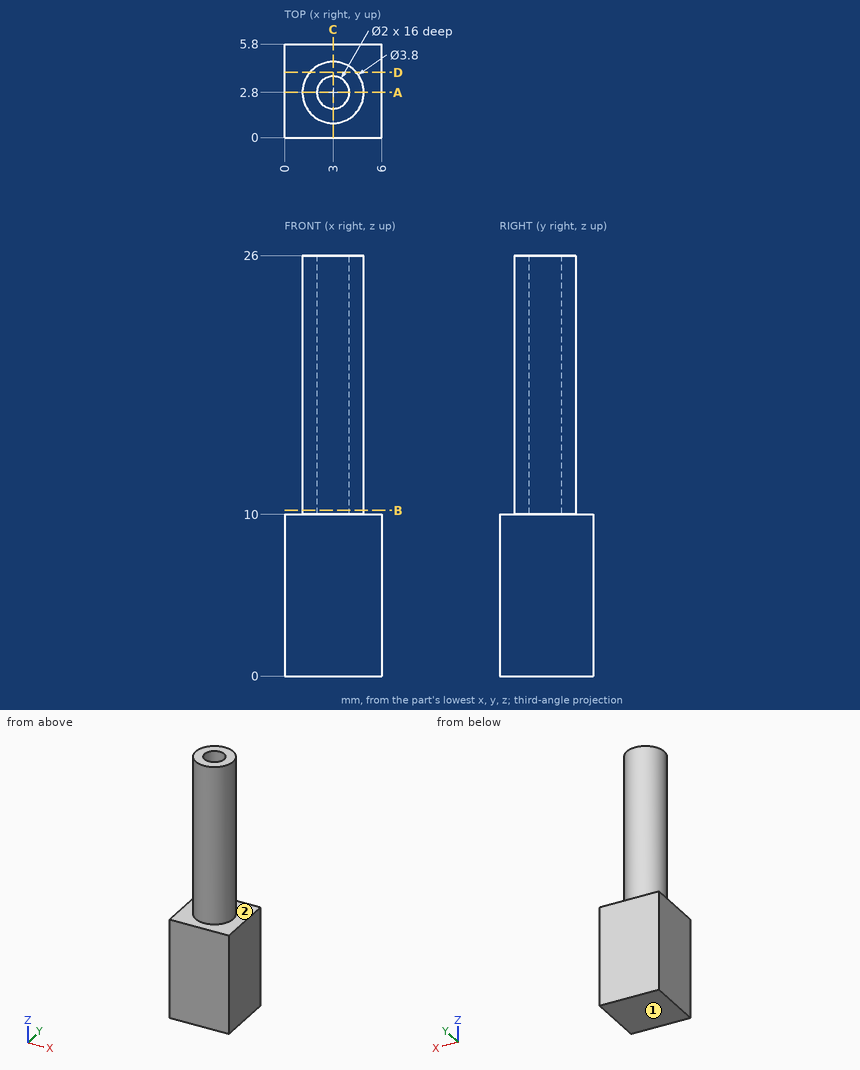
Study the drawing (mm; zero at the part's minimum x, y, z) and answer. A direction names the side the tool comes from. Give positions to 0.01 mm unless a question says otherwise; leave off trailing zeros. Order: outer loops, then holes, each group sorted by start corner. A loop starts at its lowest first (then second) coordinate and runs counter-clockwise, first axis right, second up. Notation, with made-up numbers: (62.5, 45) - (103.5, 45) arc R15 cw to (103.5, 74) - close; hole circle Ø11 at (7.5, 60). An arc over 180 degrees is marked (long way). Answer in a Markdown table with one row per item. Add a question column.
Q1. The part is cut by section A-A (y = 2.8). Determine the outline of the cut face in (x, z).
Q2. The part is cut by section D-D (y = 4.05). Determine the outline of the cut face in (x, z).
Q3. Which of the six approach directions +Z, -Z, +X, -X, +Y, -Y give full straight-line access (tool end or side, diameter ignored) to the marked faces 1 and 2?
Q4. The part is cut by section B-B (z = 10.25). Determine the outline of the cut face in (x, y), then the cut area to 3 significant figures.
Q5. Find the intervals of material crossed by line 1 along Y through (x, z) = (3.1, 13); line 2 along Z through (x, y) = (3, 3.25); line 3 along X through (y, z) = (3.5, 12.75), in increasing order. Write a range as [from, to].
Q6. The part is cut by section C-C (x = 3). Determine the outline of the cut face in (y, z).
Q7. Given P1, Ø1.8, axis at x = 3, y = 2.8, coming from the +Z side; P2, Ø1, axis at y = 3.5, z = 13, coming from the -X side, each flat-ended and moving along its own axis, determine where each tip first touches the part or whether it passes through.
Determined:
| question | item | result |
|---|---|---|
| 1 | outline | (0, 0) - (6, 0) - (6, 10) - (4.9, 10) - (4.9, 26) - (4, 26) - (4, 10) - (2, 10) - (2, 26) - (1.1, 26) - (1.1, 10) - (0, 10) - close |
| 2 | outline | (0, 0) - (6, 0) - (6, 10) - (4.43, 10) - (4.43, 26) - (1.57, 26) - (1.57, 10) - (0, 10) - close |
| 3 | face 1 | -Z, +X, -X, +Y, -Y |
| 3 | face 2 | +Z |
| 4 | outline | circle Ø3.8 at (3, 2.8); hole circle Ø2 at (3, 2.8) |
| 4 | area | 8.20 mm² |
| 5 | line 1 | y = [0.9, 1.81], [3.79, 4.7] |
| 5 | line 2 | z = [0, 10] |
| 5 | line 3 | x = [1.23, 2.29], [3.71, 4.77] |
| 6 | outline | (0, 0) - (5.8, 0) - (5.8, 10) - (4.7, 10) - (4.7, 26) - (3.8, 26) - (3.8, 10) - (1.8, 10) - (1.8, 26) - (0.9, 26) - (0.9, 10) - (0, 10) - close |
| 7 | P1 | stops at z = 10 |
| 7 | P2 | stops at x = 1.11 |
